Check sheet for the drawn part. Datum: minimum x, y, z corner. Units: mm. Round coordinates to 2 decimals unless told otherwise and drop trailing zeros. Write each loop counter-clockwise with the first axis right and the second up, starting at its lowest first coordinate (ties: lowest second). Pieces come first, ordered by that corner, then holes. Notation, with made-up numbers: (65, 45.5) - (103, 45.5) arc R20 ccw to (103, 83.5) - close; hole circle Ø10 at (-21.75, 8.25). An arc over 180 degrees is marked (long way). Answer as a JSON object with one key per item and string values. Group by question number.
1) Section check B-B (x = 8.75). Enter the section's corners in (y, z), then the cut area to 3 significant figures.
2) Go/stop test with flat-tipped pins: pin 1 Ø2 at (x, z) = (5.5, 3.5) entering from -Y; pin 2 Ø0.7 at (x, y) = (12.5, 2) entering from +Z; pin 3 Ø0.5 at (x, y) = (2, 2) entering from -Z. Record where each tip stops, or that it passes through.
3) Section check C-C (z = 2.4). Enter the section's corners in (x, y).
4) Thickness scan on line 1 (Y direction, x = 18.5, z = 1.6). Record the ranges inside material, lowest first.
5) Section check A-A (y = 2). Enter the section's corners in (x, z).
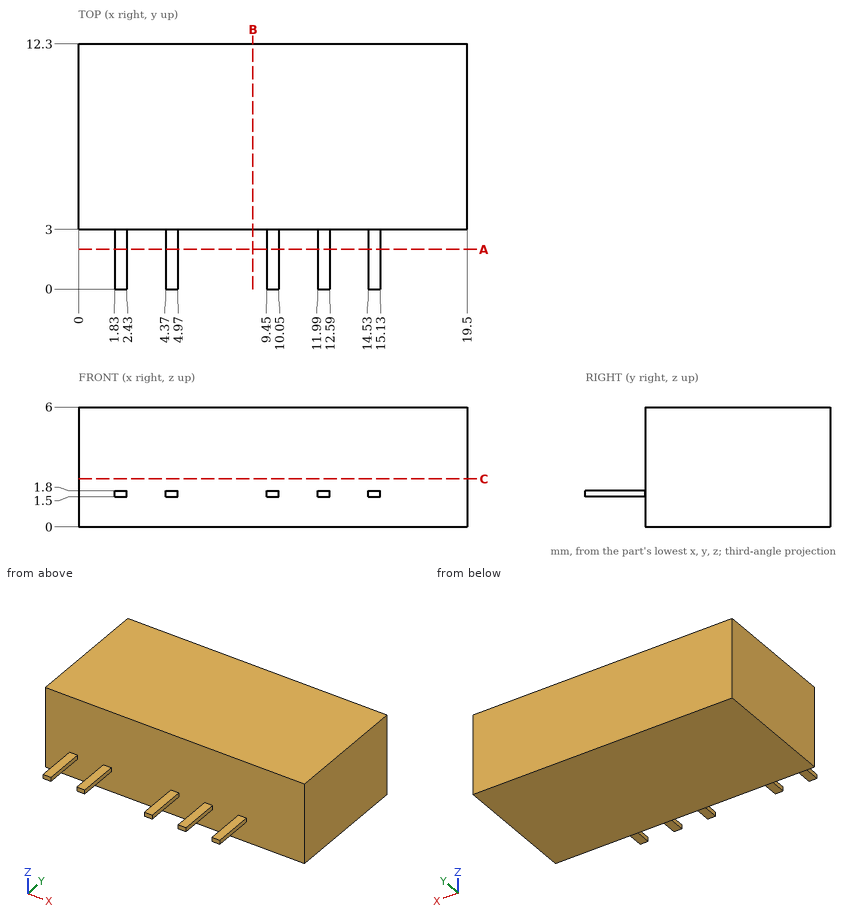
Returned:
{
 "1": {"outline": "(3, 0) - (12.3, 0) - (12.3, 6) - (3, 6) - close", "area": "55.8 mm2"},
 "2": {"pin 1": "y = 3", "pin 2": "z = 1.8", "pin 3": "z = 1.5"},
 "3": {"outline": "(0, 3) - (19.5, 3) - (19.5, 12.3) - (0, 12.3) - close"},
 "4": {"line 1": "3 to 12.3"},
 "5": {"outline": "(1.83, 1.5) - (2.43, 1.5) - (2.43, 1.8) - (1.83, 1.8) - close; (4.37, 1.5) - (4.97, 1.5) - (4.97, 1.8) - (4.37, 1.8) - close; (9.45, 1.5) - (10.05, 1.5) - (10.05, 1.8) - (9.45, 1.8) - close; (11.99, 1.5) - (12.59, 1.5) - (12.59, 1.8) - (11.99, 1.8) - close; (14.53, 1.5) - (15.13, 1.5) - (15.13, 1.8) - (14.53, 1.8) - close"}
}
